Part print with two shaded views. Sizes in mm from the minimum x, y, z corner. A direction names the side the tool comes from. Coordinates: 2 decimals unless noted, no trailing zeros. Loops run counter-clockwise (first coordinate to the right, second up) from the corner with the lowest first, then second, coordinate; pieces in that order, holes last.
(1) Two-plate mould, pull along X, no slides. Class the marked faces 1, 2, 3 and 4: pulls with the +X half, pulls with the -X half, needs draft (parallel to the pull), parting line crosses it, or undercut.
(2) Flat gauge pins, fed straight in: P1, Ø6, axis at x = 45.5, z = 7, coming from the +Y side; P2, Ø1.5, axis at y = 17, z = 6.5, coming from the -X side; P3, Ø3.5, axis at x = 74, z = 8.5, coming from the -Y side; P4, Ø4, axis at x = 6.25, z = 6, coming from the +Y side. Where does each tip first touch, or does it go through?
(3) Wall check: L1, parallel to X at y = 14, z = 10; L2, parallel to Z at x = 6.25, y = 45.7; L3, parallel to X at y = 45, z = 11. Give the ranges that are in metal, low to high.
(4) Slice it at D-D (z = 10.25). Give the cut face in (x, y).
(5) Slice it at B-B (z = 6). Give the cut face in (x, y).
(6) Slice it at C-C (x = 74.75). Give the cut face in (y, z).
(7) Slice it at A-A (y = 19.5). Give the cut face in (x, z), and give its area (3 significant figures).
(8) Tool access for the marked faces 5, 6 and 7: list every direction of +Z, -Z, +X, -X, +Y, -Y with a clear straight run to the whole face (end or side of a thin tool).
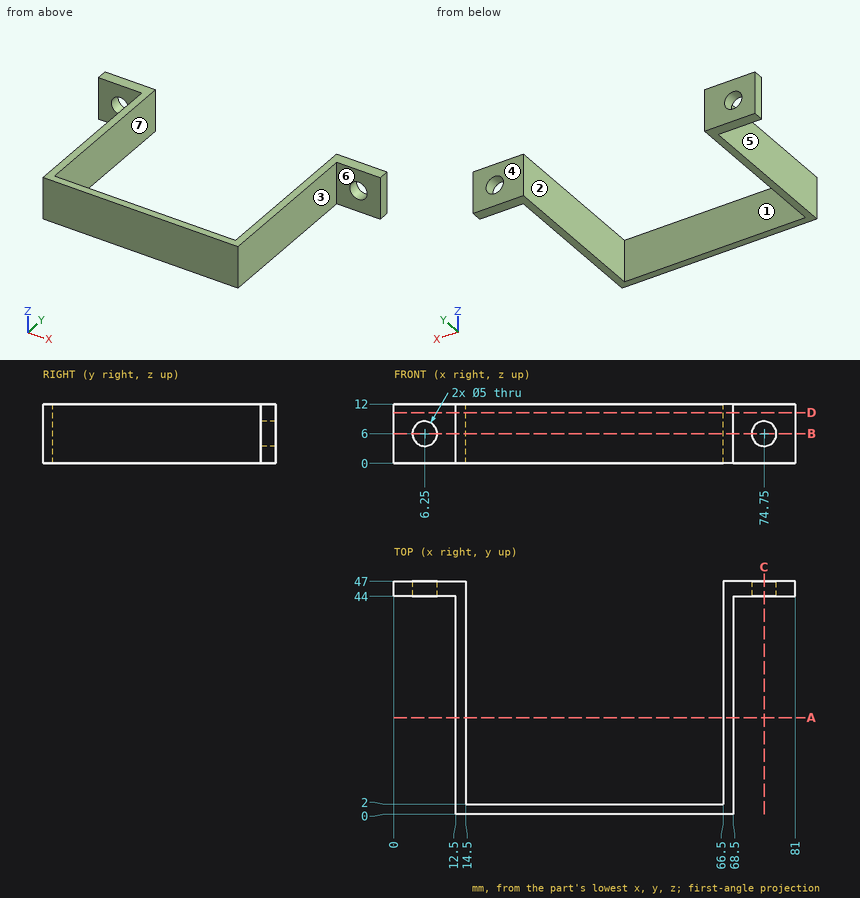
Response values:
1. face 1: undercut
1. face 2: undercut
1. face 3: pulls with the +X half
1. face 4: needs draft
2. P1: stops at y = 2
2. P2: stops at x = 12.5
2. P3: stops at y = 44
2. P4: passes through
3. L1: x = 12.5 to 14.5, 66.5 to 68.5
3. L2: z = 0 to 3.5, 8.5 to 12
3. L3: x = 0 to 14.5, 66.5 to 81
4. outline: (0, 44) - (12.5, 44) - (12.5, 0) - (68.5, 0) - (68.5, 44) - (81, 44) - (81, 47) - (66.5, 47) - (66.5, 2) - (14.5, 2) - (14.5, 47) - (0, 47) - close
5. outline: (0, 44) - (3.75, 44) - (3.75, 47) - (0, 47) - close; (8.75, 44) - (12.5, 44) - (12.5, 0) - (68.5, 0) - (68.5, 44) - (72.25, 44) - (72.25, 47) - (66.5, 47) - (66.5, 2) - (14.5, 2) - (14.5, 47) - (8.75, 47) - close; (77.25, 44) - (81, 44) - (81, 47) - (77.25, 47) - close
6. outline: (44, 0) - (47, 0) - (47, 3.5) - (44, 3.5) - close; (44, 8.5) - (47, 8.5) - (47, 12) - (44, 12) - close
7. outline: (12.5, 0) - (14.5, 0) - (14.5, 12) - (12.5, 12) - close; (66.5, 0) - (68.5, 0) - (68.5, 12) - (66.5, 12) - close
7. area: 48.0 mm2
8. face 5: +Z, -Z, -X, -Y
8. face 6: +Z, -Z, +X, -Y
8. face 7: +Z, -Z, +Y
